from build123d import *

# Parameters (mm, degrees)
F0_R          = 70
F0_R_2        = 65
F1_DEPTH      = 1334
F2_W          = 200
F2_H          = 200
F2_R          = 11
F3_DEPTH      = 10
F4_W          = 30.1787997812
F4_H          = 10
F4_W_2        = 10
F4_H_2        = 30.1787997812
F5_DEPTH      = 150
F6_T1_DEPTH   = 269.311363913
F6_T3_DEPTH   = 269.311363913
F6_T8_DEPTH   = 269.311363913
F6_S9_R       = 70
F6_T10_DEPTH  = 139
F8_W          = 200
F8_H          = 200
F8_R          = 8.5
F9_DEPTH      = 10
F10_W         = 10
F10_H         = 30.1787997812
F10_W_2       = 30.1787997812
F10_H_2       = 10
F11_DEPTH     = 80
F12_T1_DEPTH  = 269.311363913
F12_T3_DEPTH  = 269.311363913
F12_T8_DEPTH  = 269.311363913
F12_S9_R      = 70
F12_T10_DEPTH = 139
F12_T14_DEPTH = 269.311363913
F12_S15_R     = 70
F12_T16_DEPTH = 139


# Not quite as in the source:
# - a fillet or chamfer that OpenCascade refuses, or shapes differently, is made with other operations: its cross-section is extruded or revolved along the edge and cut away or added


with BuildPart() as f1:
    # F0 (on Front) → F1 (new body)
    with BuildSketch(Plane.XZ):
        Circle(F0_R)
        Circle(F0_R_2, mode=Mode.SUBTRACT)
    extrude(amount=F1_DEPTH)

    # F2 (on Front) → F3 (join)
    with BuildSketch(Plane.XZ):
        Rectangle(F2_W, F2_H)
        with Locations((-75, -75)):
            Circle(F2_R, mode=Mode.SUBTRACT)
        with Locations((75, -75)):
            Circle(F2_R, mode=Mode.SUBTRACT)
        with Locations((-75, 75)):
            Circle(F2_R, mode=Mode.SUBTRACT)
        with Locations((75, 75)):
            Circle(F2_R, mode=Mode.SUBTRACT)
    extrude(amount=-F3_DEPTH)

    # F4 (on Front) → F5 (join)
    with BuildSketch(Plane.XZ):
        with Locations((-84.9106001094, 0)):
            Rectangle(F4_W, F4_H)
        with Locations((0, 84.9106001094)):
            Rectangle(F4_W_2, F4_H_2)
        with Locations((84.9106001094, 0)):
            Rectangle(F4_W, F4_H)
        with Locations((0, -84.9106001094)):
            Rectangle(F4_W_2, F4_H_2)
    extrude(amount=F5_DEPTH)

    # F6: chamfer of 50 x 20 on 4 edges, made by hand

    # F6_s2 → F6_t1 (cut)
    with BuildSketch(Plane.YZ.offset(-134.6556819565)):
        Polygon((-100, 100), (-150, 80), (-150, 100), align=None)
        Polygon((-100, -100), (-150, -80), (-150, -100), align=None)
    extrude(amount=F6_T1_DEPTH, mode=Mode.SUBTRACT)

    # F6_s4 → F6_t3 (cut)
    with BuildSketch(Plane.XY.offset(-134.6556819565)):
        Polygon((100, -100), (80, -150), (100, -150), align=None)
    extrude(amount=F6_T3_DEPTH, mode=Mode.SUBTRACT)


with BuildPart() as f6_tool6:
    # F6_s7 → F6_t8 (new body)
    with BuildSketch(Plane.XY.offset(134.6556819565)):
        Polygon((-100, -130), (-50, -150), (-100, -150), align=None)
    extrude(amount=-F6_T8_DEPTH)

    # F6_s9 → F6_t10 (cut, symmetric)
    with BuildSketch(Plane.XZ.offset(140)):
        Circle(F6_S9_R)
    extrude(amount=F6_T10_DEPTH, both=True, mode=Mode.SUBTRACT)


with BuildPart() as f1_1:
    add(f1.part)

    # F6_t5: cut F6_tool6
    add(f6_tool6.part, mode=Mode.SUBTRACT)

    # F8 (on offset) → F9 (join)
    with BuildSketch(Plane.XZ.offset(1334)):
        Rectangle(F8_W, F8_H)
        with Locations((-75, -75)):
            Circle(F8_R, mode=Mode.SUBTRACT)
        with Locations((75, -75)):
            Circle(F8_R, mode=Mode.SUBTRACT)
        with Locations((-75, 75)):
            Circle(F8_R, mode=Mode.SUBTRACT)
        with Locations((75, 75)):
            Circle(F8_R, mode=Mode.SUBTRACT)
    extrude(amount=F9_DEPTH)

    # F10 (on face) → F11 (join)
    with BuildSketch(Plane(origin=(0, -1334, 0), x_dir=(-1, 0, 0), z_dir=(0, 1, 0))):
        with Locations((0, 84.9106001094)):
            Rectangle(F10_W, F10_H)
        with Locations((84.9106001094, 0)):
            Rectangle(F10_W_2, F10_H_2)
        with Locations((0, -84.9106001094)):
            Rectangle(F10_W, F10_H)
        with Locations((-84.9106001094, 0)):
            Rectangle(F10_W_2, F10_H_2)
    extrude(amount=F11_DEPTH)

    # F12: chamfer of 20 x 50 on 4 edges, made by hand

    # F12_s2 → F12_t1 (cut)
    with BuildSketch(Plane.YZ.offset(-134.6556819565)):
        Polygon((-1304, 100), (-1254, 80), (-1254, 100), align=None)
    extrude(amount=F12_T1_DEPTH, mode=Mode.SUBTRACT)

    # F12_s4 → F12_t3 (cut)
    with BuildSketch(Plane.XY.offset(-134.6556819565)):
        Polygon((100, -1304), (80, -1254), (100, -1254), align=None)
    extrude(amount=F12_T3_DEPTH, mode=Mode.SUBTRACT)


with BuildPart() as f12_tool6:
    # F12_s7 → F12_t8 (new body)
    with BuildSketch(Plane.XY.offset(-134.6556819565)):
        Polygon((-100, -1274), (-50, -1254), (-100, -1254), align=None)
    extrude(amount=F12_T8_DEPTH)

    # F12_s9 → F12_t10 (cut, symmetric)
    with BuildSketch(Plane.XZ.offset(1264)):
        Circle(F12_S9_R)
    extrude(amount=F12_T10_DEPTH, both=True, mode=Mode.SUBTRACT)


with BuildPart() as f1_2:
    add(f1_1.part)

    # F12_t5: cut F12_tool6
    add(f12_tool6.part, mode=Mode.SUBTRACT)


with BuildPart() as f12_tool12:
    # F12_s13 → F12_t14 (new body)
    with BuildSketch(Plane.YZ.offset(134.6556819565)):
        Polygon((-1274, -100), (-1254, -50), (-1254, -100), align=None)
    extrude(amount=-F12_T14_DEPTH)

    # F12_s15 → F12_t16 (cut, symmetric)
    with BuildSketch(Plane.XZ.offset(1264)):
        Circle(F12_S15_R)
    extrude(amount=F12_T16_DEPTH, both=True, mode=Mode.SUBTRACT)


with BuildPart() as f1_3:
    add(f1_2.part)

    # F12_t11: cut F12_tool12
    add(f12_tool12.part, mode=Mode.SUBTRACT)


solid = f1_3.part
Input: part model. Units: mm. Frame: model coordinates. A direction names the side the tool comes from. Give positions to 0.01 mm unless a question says otherwise; leave off trailing zeros. Loops run counter-clockwise (first coordinate to the right, second up) from the corner with the lowest first, then second, coordinate; pieces in that order, holes last. Notation, with made-up numbers: M 63.25,26 L 107.25,26 A29 ccw 107.25,61 Z; hole C 76,41 d4. An arc over 180 degrees is marked long. Use one line per item in the form item = value.
1. Line query: L1, parallel to Z at x = 75, y = -1336.75; L2, parallel to Z at x = -75, y = 6; L3, parallel to Y at x = 35, z = 41.5. Output: solid intervals per line, ascending.
Numbers:
L1 = -100 to -83.5, -66.5 to 66.5, 83.5 to 100
L2 = -100 to -86, -64 to 64, 86 to 100
L3 = -1344 to -1334, 0 to 10
2. Section query C-C, the plane y = -938. Return the cut outline in (x, z).
Numbers:
outline = C 0,0 d140; hole C 0,0 d130
3. First-contact query: pin 1 (12 mm diameter, centred on y = -162.5, z = -70.5, fed in from +X); pin 2 (15 mm diameter, centred on x = 82, y = -1284.5, fed in from +Z); pin 3 (5 mm diameter, centred on y = -1030.5, z = -32.5, fed in from +X). Flat tips, straight axial feed; report the tip coordinate or a pass-through.
Numbers:
pin_1 = 27.2
pin_2 = 5
pin_3 = 63.25
4. Reachability of faces 4 (the face through (-64, 0, -62)), 5 (the face through (73.568, 4.93, 85.906)), 6 (the face through (-5, -74, 85)), 7 (the face through (82, -1303, -5)) from +Z, -Z, +X, -X, +Y, -Y: full face, straight path, thin tool, end or side. Return the list, or none.
Numbers:
face_4 = -Z, -X
face_5 = +Y
face_6 = +Z, -X
face_7 = -Z, +X
5. Section query A-A, the plane x = 35.5. Return the cut outline in (y, z), and give its area (3 significant figures).
Numbers:
outline = M -1344,-100 L -1334,-100 L -1334,-60.33 L 0,-60.33 L 0,-100 L 10,-100 L 10,100 L 0,100 L 0,60.33 L -1334,60.33 L -1334,100 L -1344,100 Z; hole M -1334,-54.45 L 0,-54.45 L 0,54.45 L -1334,54.45 Z
area = 19,700 mm²
6. Pull-direction query (X, two-part tool) for faces 1 (the face through (62, -657.66, 19.52)), 2 (the face through (64.662, -657.662, -26.81)), 3 (the face through (62, 0, 64)); classes: released by +X, released by -X, zero draft, split by the parting line, or undercut.
Numbers:
face_1 = undercut
face_2 = split by the parting line
face_3 = zero draft
7. Section query B-B, the plane z = -31. Return the cut outline in (x, y), and give its area (3 significant figures).
Numbers:
outline = M -100,-1344 L 100,-1344 L 100,-1334 L 62.76,-1334 L 62.76,0 L 100,0 L 100,10 L -100,10 L -100,0 L -62.76,0 L -62.76,-1334 L -100,-1334 Z; hole M -57.13,-1334 L 57.13,-1334 L 57.13,0 L -57.13,0 Z
area = 19,000 mm²
